Autodesk Inventor part; units mm, degrees
ref_plane "YZ Plane" through (0, 0, 0) normal (1, 0, 0) x (0, 1, 0)
ref_plane "XZ Plane" through (0, 0, 0) normal (0, 1, 0) x (-1, 0, 0)
ref_plane "XY Plane" through (0, 0, 0) normal (0, 0, 1) x (1, 0, 0)
sketch "スケッチ1" plane through (0, 0, 0) normal (0, 0, 1) x (1, 0, 0)
  circle A0 centre (0, 0) radius 4
  dimension "d13" = 8
extrude "押し出し1" add sketch "スケッチ1" along normal mid plane 45
sketch "スケッチ2" plane through (0, 0, 22.5) normal (0, 0, 1) x (1, 0, 0)
  point P0 (0, 0)
  point P1 (0, 0)
hole "穴1" at (0, 0, 22.5) direction (0, 0, -1) diameter 3.242 depth 11.8 tip angle 118
mirror "ミラー1" about plane through (0, 0, 0) normal (0, 0, 1) of "穴1"
chamfer "面取り1" distance 0.2 angle 45 4 edges at (0, 1.621, 22.5) (-4, 0, 22.5) (-4, 0, -22.5) (0, 1.621, -22.5)
properties part number "ARF-445" material "鋼、炭素鋼"
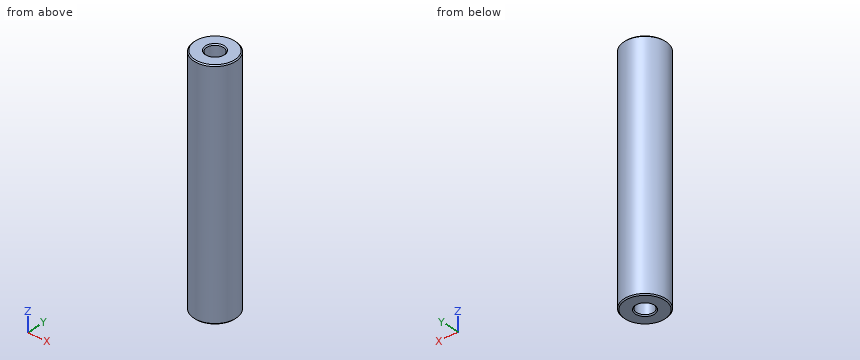
Design review of the part built by this model. Coordinates are the model's own, in mm. Give positions to 0.01 mm unless a question says otherwise; leave off trailing zeros. Loops run counter-clockwise (first coordinate to the right, second up) from the corner with the lowest first, then second, coordinate; pieces in that order, holes last. Notation, with made-up numbers: M -40,-19 L -20,-19 A21 cw -20,0 Z; hole C 9,88.25 d3. An arc over 180 degrees is marked long. Answer as a JSON object with one key per item and string values.
Item 1: For P1, Ø1.9, axis at x = 0, y = 0, coming from the +Z side; P2, Ø1, axis at x = -2, z = 5.5, coming from the +Y side; P3, Ø1, axis at y = -2, z = -15, coming from the +X side, all flat-tipped, find the tip position at first contact; note any pin that passes through.
Output values:
{"P1": "stops at z = 10.3", "P2": "stops at y = 3.71", "P3": "stops at x = 3.71"}
Item 2: We need section A-A (z = 14). State the section outline as (x, y) points.
Output values:
{"outline": "C 0,0 d8; hole C 0,0 d3.24"}
Item 3: Wall thickness on line 1 along Y through (x, z) = (0, 15.25); line 2 along Y through (x, z) = (1.25, 1.5): over which ranges is each line inside the solid? List them lowest first.
Output values:
{"line 1": "y = -4 to -1.62, 1.62 to 4", "line 2": "y = -3.8 to 3.8"}
Item 4: We need section B-B (z = 6.5). State the section outline as (x, y) points, and give its area (3 significant figures).
Output values:
{"outline": "C 0,0 d8", "area": "50.3 mm2"}
